Geometry: final body of the model. Coordinates: model frame, mm. A direction names the side the tool comes from. Give positions to 0.01 mm unless a question says otherwise; leave off trailing zeros. Write each loop counter-clockwise with the first axis right and the second up, starting at its lowest first coordinate (ties: lowest second). Pieces come first, ordered by that corner, then holes.
```python
from build123d import *

# Parameters (mm, degrees)
F1_DEPTH = 30
F2_R     = 30
F3_DEPTH = 10
F4_R     = 30
F5_DEPTH = 10


# Not quite as in the source:
# - ends of sketch curves that miss each other by under 0.0002 mm in the source are joined


with BuildPart() as f1:
    # F0 (on Top) → F1 (new body)
    with BuildSketch(Plane.XY):
        with BuildLine():
            Line((-83.6328645892, 0), (-83.6328645892, -25))
            Line((-83.6328645892, -25), (-74.6328645685, -25))
            Line((-74.6328645685, -25), (-74.6328645685, 0))
            ThreePointArc((-74.6328645685, 0), (-72.9577352395, 4.1587851122), (-68.8677000121, 5.9954025783))
            Line((-68.8677000121, 5.9954025783), (80.9957853142, 5.9954025783))
            ThreePointArc((80.9957853142, 5.9954025783), (85.2384259867, 4.2380432715), (86.9957852935, -0.004597401))
            Line((86.9957852935, -0.004597401), (86.9957845889, -25))
            Line((86.9957845889, -25), (95.9957846097, -25))
            Line((95.9957846097, -25), (95.9957846097, 0))
            ThreePointArc((95.9957846097, 0), (91.6007614807, 10.603629619), (80.9957853142, 14.995402599))
            Line((80.9957853142, 14.995402599), (-69.0042146858, 14.995402599))
            ThreePointArc((-69.0042146858, 14.995402599), (-79.3699557095, 10.4744868264), (-83.6328645892, 0))
        make_face()
    extrude(amount=F1_DEPTH)

    # F2 (on face) → F3 (join)
    with BuildSketch(Plane.XZ.offset(25)):
        with Locations((-79.1328645789, 15)):
            Circle(F2_R)
    extrude(amount=F3_DEPTH)

    # F4 (on face) → F5 (join)
    with BuildSketch(Plane.XZ.offset(25)):
        with Locations((91.4957845993, 15)):
            Circle(F4_R)
    extrude(amount=F5_DEPTH)


solid = f1.part
```
Item 1: Section C-C, the plane z = 15. Return the cut outline in (x, y), plus the area to 3 significant figures.
Found:
outline: (-109.13, -35) - (-49.13, -35) - (-49.13, -25) - (-74.63, -25) - (-74.63, 0) arc R6 cw to (-68.87, 6) - (81, 6) arc R6 cw to (87, 0) - (87, -25) - (61.5, -25) - (61.5, -35) - (121.5, -35) - (121.5, -25) - (96, -25) - (96, 0) arc R15 ccw to (81, 15) - (-69, 15) arc R15 ccw to (-83.63, 0) - (-83.63, -25) - (-109.13, -25) - close
area: 3,290 mm2
Item 2: Reachability of faces 4 (the face through (-101.24, -29.93, 35.28)), 5 (the face through (6, 8, 0)), 6 (the face through (95.996, -13, 15)), 7 (the face through (5, 5.995, 15)), 8 (the face through (-83.633, -12, 15)) from +Z, -Z, +X, -X, +Y, -Y: full face, straight path, thin tool, end or side. Return the list, or none.
Found:
face 4: -Y
face 5: -Z, +X, -X, +Y
face 6: +Z, -Z, +X, +Y
face 7: +Z, -Z
face 8: +Z, -Z, -X, +Y
Item 3: Pin query (flat end, axial travel): pin 1 Ø12 at (y, z) = (8, 0) entering from -X; pin 2 Ø20 at (y, z) = (-10, 19.5) entering from -X; pin 3 Ø3 at (x, y) = (83.5, -21) entering from +Z; pin 4 Ø20 at (y, z) = (-8, 12) entering from +X. Return the tip coordinate at first contact, or that it passes through.
Found:
pin 1: stops at x = -83.5
pin 2: stops at x = -83.63
pin 3: passes through
pin 4: stops at x = 96
Item 4: Line query: L1, parallel to X at y = -13, z = 4.5; L2, parallel to Y at x = -24, z = 22; L3, parallel to X at y = 2, z = 4.5. Output: solid intervals per line, ascending.
Found:
L1: x = -83.63 to -74.63, 87 to 96
L2: y = 6 to 15
L3: x = -83.5 to -74.29, 86.65 to 95.86
Item 5: Section A-A, the plane y = -15. Return the cut outline in (x, z).
Found:
outline: (-83.63, 0) - (-74.63, 0) - (-74.63, 30) - (-83.63, 30) - close; (87, 0) - (96, 0) - (96, 30) - (87, 30) - close
Item 6: Section D-D, the plane x = 89.5. Return the cut outline in (y, z), plus the area to 3 significant figures.
Found:
outline: (-35, -14.93) - (-25, -14.93) - (-25, 0) - (12.35, 0) - (12.35, 30) - (-25, 30) - (-25, 44.93) - (-35, 44.93) - close
area: 1,720 mm2
Item 7: Section B-B, the plane x = 66. Return the cut outline in (y, z).
Found:
outline: (-35, -0.81) - (-25, -0.81) - (-25, 30.81) - (-35, 30.81) - close; (6, 0) - (15, 0) - (15, 30) - (6, 30) - close
Item 8: Pull-direction query (Y, two-part tool) for faces 1 (the face through (-73.002, 4.112, 14.79)), 2 (the face through (6, 8, 30)), 3 (the face through (-80, -35, 15)); classes: +Y half, -Y half, draft (parallel to the pull), parting line (faces both ways), or undercut.
Found:
face 1: undercut
face 2: draft
face 3: -Y half
